Model file for the job. Use its own axes, mm. A direction names the side the tool comes from. Round coordinates to 2 decimals unless told otherwise and drop trailing zeros. Order: outer loops, then holes, each group sorted by start corner. A loop starts at its lowest first (then second) coordinate and runs counter-clockwise, first axis right, second up. Notation, with made-up numbers: M 89,-4 L 127,-4 A19 cw 127,14 Z; hole C 86,28 d8. An arc over 180 degrees is marked long. Return JSON: item names as keys, results as strings. Group by question number.
Item 1: Slice it at D-D on x = -79. Write the cut outline in (y, z).
Item 2: Which spindle directions (+Z, -Z, +X, -X, +Y, -Y) get a long thin tool onto all of the face, cutting with end or side? Do faces 1 (the face through (59, -19, 5)), 2 (the face through (-67.6, -2.2, 2.5)). Say none if no direction does.
Item 3: Probe line 1 along Y through (x, z) = (0, 3.3); line 2 along Y through (x, z) = (0, 1.1); line 3 along Y through (x, z) = (-30, 4.4). List the from-to ranges inside material, lowest first.
Item 4: Pin check, flat tips, straight feed: pin 1 Ø5 at (x, y) = (-1, -69.5) entering from +Z; pin 2 Ø1 at (x, z) = (-21.5, 4) entering from +Y. Stop position of each tip, or through.
Item 5: Slice it at B-B on z = 0.95. Write the cut outline in (x, y).
Item 6: Slice it at C-C on x = -37. Write the cut outline in (y, z).
Item 7: Slice it at A-A on y = -30. Write the cut outline in (x, z), then the cut area to 3 significant figures.
from build123d import *

# Parameters (mm, degrees)
SKETCH_R     = 90
SKETCH_R_2   = 60.75
SKETCH_R_3   = 2
PAD_DEPTH    = 5
SKETCH001_R  = 5
POCKET_DEPTH = 2.5


with BuildPart() as part:
    # Sketch → Pad (new body)
    with BuildSketch(Plane.XY):
        Circle(SKETCH_R)
        Circle(SKETCH_R_2, mode=Mode.SUBTRACT)
        with Locations((0, 67.5)):
            Circle(SKETCH_R_3, mode=Mode.SUBTRACT)
        with Locations((67.5, 0)):
            Circle(SKETCH_R_3, mode=Mode.SUBTRACT)
        with Locations((0, -67.5)):
            Circle(SKETCH_R_3, mode=Mode.SUBTRACT)
        with Locations((-67.5, 0)):
            Circle(SKETCH_R_3, mode=Mode.SUBTRACT)
        with Locations((-58.336309, -58.336309)):
            Circle(SKETCH_R_3, mode=Mode.SUBTRACT)
        with Locations((58.336309, 58.336309)):
            Circle(SKETCH_R_3, mode=Mode.SUBTRACT)
    extrude(amount=PAD_DEPTH)

    # Sketch001 (on Face10 of Pad) → Pocket (cut)
    with BuildSketch(Plane.XY.offset(5)):
        with Locations((67.5, 0)):
            Circle(SKETCH001_R)
        with Locations((0, 67.5)):
            Circle(SKETCH001_R)
        with Locations((-67.5, 0)):
            Circle(SKETCH001_R)
        with Locations((0, -67.5)):
            Circle(SKETCH001_R)
    extrude(amount=-POCKET_DEPTH, mode=Mode.SUBTRACT)


solid = part.part
Output values:
{
 "1": {"outline": "M -43.12,0 L 43.12,0 L 43.12,5 L -43.12,5 Z"},
 "2": {"face 1": "+Z, +X, -X, +Y, -Y", "face 2": "+Z"},
 "3": {"line 1": "-90 to -72.5, -62.5 to -60.75, 60.75 to 62.5, 72.5 to 90", "line 2": "-90 to -69.5, -65.5 to -60.75, 60.75 to 65.5, 69.5 to 90", "line 3": "-84.85 to -52.83, 52.83 to 84.85"},
 "4": {"pin 1": "z = 2.5", "pin 2": "y = 87.52"},
 "5": {"outline": "C 0,0 d180; hole C -67.5,0 d4; hole C 0,0 d121.5; hole C -58.34,-58.34 d4; hole C 0,-67.5 d4; hole C 0,67.5 d4; hole C 58.34,58.34 d4; hole C 67.5,0 d4"},
 "6": {"outline": "M -82.04,0 L -48.18,0 L -48.18,5 L -82.04,5 Z; M 48.18,0 L 82.04,0 L 82.04,5 L 48.18,5 Z"},
 "7": {"outline": "M -84.85,0 L -52.83,0 L -52.83,5 L -84.85,5 Z; M 52.83,0 L 84.85,0 L 84.85,5 L 52.83,5 Z", "area": "320 mm²"}
}
